Verification items for the finished model (mm, model axes). Face numbers are marked on the shaded views. A direction names the side the tool comes from. Coordinates: 2 decimals unless noted, no trailing zeros. Write each loop counter-clockwise with the first axis right and the second up, starting at its lowest first coordinate (ties: lowest second). Pieces come first, ordered by that corner, then holes. Notation, with made-up numbers: (78.25, 42.5) -> (117.25, 42.5) arc R33 ccw to (117.25, 74.5) -> close; hole circle Ø9 at (51.5, -26). An arc over 180 degrees is marked (long way). Use CSV: the item, a comma, the result in double quotes.
```python
from build123d import *

# Parameters (mm, degrees)
PAD_DEPTH    = 4.5
CHAMFER_SIZE = 1
FILLET_R     = 1
FILLET001_R  = 0.75
FILLET002_R  = 6
FILLET003_R  = 1


with BuildPart() as part:
    # Sketch → Pad (new body)
    with BuildSketch(Plane.XY):
        Polygon((0, 0), (0, 8), (14.4, 8), (14.4, 5.4), (13.4, 3.786999), (12.6, 3.786999), (12.6, 6.2), (1.8, 6.2), (1.8, 1.8), (14.2, 1.8), (14.2, 2.8), (15.2, 4.413001), (16, 4.413001), (16, 0), align=None)
    extrude(amount=PAD_DEPTH)

    # Chamfer
    chamfer_edges = [part.edges().sort_by_distance(p)[0] for p in [
        (0, 8, 2.25),
        (0, 0, 2.25),
        (16, 0, 2.25),
    ]]
    chamfer(chamfer_edges, length=CHAMFER_SIZE)

    # Fillet
    fillet_edges = [part.edges().sort_by_distance(p)[0] for p in [
        (1.8, 6.2, 2.25),
        (1.8, 1.8, 2.25),
        (12.6, 6.2, 2.25),
    ]]
    fillet(fillet_edges, radius=FILLET_R)

    # Fillet001
    fillet001_edges = [part.edges().sort_by_distance(p)[0] for p in [
        (14.2, 1.8, 2.25),
    ]]
    fillet(fillet001_edges, radius=FILLET001_R)

    # Fillet002
    fillet002_edges = [part.edges().sort_by_distance(p)[0] for p in [
        (14.4, 5.4, 2.25),
    ]]
    fillet(fillet002_edges, radius=FILLET002_R)

    # Fillet003
    fillet003_edges = [part.edges().sort_by_distance(p)[0] for p in [
        (14.4, 8, 2.25),
    ]]
    fillet(fillet003_edges, radius=FILLET003_R)


solid = part.part
```
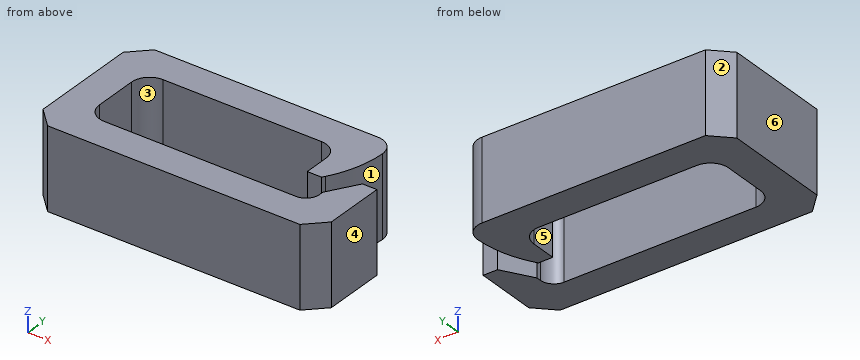
1) Scan lines: L1, parallel to Y at x = 3, z = 0.5; L2, parallel to X at y = 3.5, z = 1.75; L3, parallel to X at y = 2.5, z = 4.3. Record each from-to range of solid material in increasing order.
Return value:
L1,"0 to 1.8, 6.2 to 8"
L2,"0 to 1.8, 14.63 to 16"
L3,"0 to 1.85, 14.2 to 16"
2) Mould release check, pull along X, two halves, no side actions. Record for the marked faces 3, 4, 5 and 6: released by +X, released by -X, zero draft, split by the parting line, or undercut.
Return value:
face 3,"undercut"
face 4,"released by +X"
face 5,"undercut"
face 6,"released by -X"
3) Gauge pin test, flat ends, axial feed: pin 1 (1 mm diameter, centred on y = 5, z = 2.5, fed in from +X); pin 2 (3 mm diameter, centred on x = 10, y = 6, fed in from +Z); pin 3 (0.6 mm diameter, centred on x = 15.5, z = 1.5, fed in from +Y). Record the tip position at first contact, or that the pin passes through.
Return value:
pin 1,"x = 14.18"
pin 2,"z = 4.5"
pin 3,"y = 4.41"
4) Cross-section at C-C (y = 4.25). Record the boundary of the cut face in (x, z), plus the area to 3 significant figures.
Return value:
outline,"(0, 0) -> (1.8, 0) -> (1.8, 4.5) -> (0, 4.5) -> close; (12.6, 0) -> (13.68, 0) -> (13.68, 4.5) -> (12.6, 4.5) -> close; (15.1, 0) -> (16, 0) -> (16, 4.5) -> (15.1, 4.5) -> close"
area,"17.0 mm2"
5) Set-up check for the marked faces 1 and 2: record each of +Z, -Z, +X, -X, +Y, -Y from which the full face is reachable in a straight line by a thin tool's end or side.
Return value:
face 1,"+Z, -Z"
face 2,"+Z, -Z, -X, +Y"
6) Cross-section at A-A (x = 8.5). Record the boundary of the cut face in (y, z).
Return value:
outline,"(0, 0) -> (1.8, 0) -> (1.8, 4.5) -> (0, 4.5) -> close; (6.2, 0) -> (8, 0) -> (8, 4.5) -> (6.2, 4.5) -> close"
7) Cross-section at B-B (y = 2). Record the boundary of the cut face in (x, z).
Return value:
outline,"(0, 0) -> (2.2, 0) -> (2.2, 4.5) -> (0, 4.5) -> close; (13.96, 0) -> (16, 0) -> (16, 4.5) -> (13.96, 4.5) -> close"
